from build123d import *


with BuildPart() as part:
    # Sketch5 → Revolve2 (revolve)
    with BuildSketch(Plane.XY):
        with BuildLine():
            ThreePointArc((6.647472776, -0.637932427), (6.425260177, 0.01668478), (6.35, 0.703880554))
            Line((6.35, 0.703880554), (6.35, 5.034871939))
            ThreePointArc((6.35, 5.034871939), (6.591682484, 6.249891837), (7.27993597, 7.27993597))
            Line((7.27993597, 7.27993597), (26.9875, 26.9875))
            Line((26.9875, 26.9875), (30.1625, 26.9875))
            Line((30.1625, 26.9875), (30.1625, -51.066071045))
            Line((30.1625, -51.066071045), (6.647472776, -0.637932427))
        make_face()
        with BuildLine():
            ThreePointArc((3.175, 5.034871939), (3.416682484, 6.249891837), (4.10493597, 7.27993597))
            Line((4.10493597, 7.27993597), (23.8125, 26.9875))
            Line((23.8125, 26.9875), (26.9875, 26.9875))
            Line((26.9875, 26.9875), (7.27993597, 7.27993597))
            ThreePointArc((7.27993597, 7.27993597), (6.591682484, 6.249891837), (6.35, 5.034871939))
            Line((6.35, 5.034871939), (6.35, 0.703880554))
            ThreePointArc((6.35, 0.703880554), (6.425260177, 0.01668478), (6.647472776, -0.637932427))
            Line((6.647472776, -0.637932427), (30.1625, -51.066071045))
            Line((30.1625, -51.066071045), (26.9875, -51.066071045))
            Line((26.9875, -51.066071045), (3.472472776, -0.637932427))
            ThreePointArc((3.472472776, -0.637932427), (3.250260177, 0.01668478), (3.175, 0.703880554))
            Line((3.175, 0.703880554), (3.175, 5.034871939))
        make_face()
    revolve(axis=Axis((0, 0, 0), (0, -1, 0)))


solid = part.part
Check sheet for the modelled part. Datum: model origin and axes. Units: mm. Give positions to 0.01 mm unless a question says otherwise; leave off trailing zeros. Write each loop counter-clockwise with the first axis right and the second up, starting at its lowest first coordinate (ties: lowest second). Pieces come first, ordered by that corner, then holes. Notation, with made-up numbers: (68.5, 35.25) -> (99.5, 35.25) arc R21 ccw to (99.5, 49.25) -> close; hole circle Ø4 at (52, -23). An arc over 180 degrees is marked (long way). One line per item, written item: value. Start each with the question number.
Item 1: Material ranges on probe 1 along Z at (x, y) = (0, 1) (1 decimal); probe 2 along Y at (x, z) = (-1, -13); probe 3 along Z at (x, y) = (-23, -20), recorded low to high. Write a range as from..to.
Item 2: Draft check along X on faces 1 (the cylindrical face through (-30.133, -12.586, 1.326)), 2 (the conical face through (-9.88, -19.9, -7.58)), 3 (the flat face through (22.2, 26.988, 9.1)). Enter one of: +X half, -X half, draft (parallel to the pull), parting line (faces both ways), or undercut.
Item 3: Section check C-C on y = -7. Record the cut outline in (x, z) (1 decimal).
Item 4: Gauge pin test, flat ends, axial feed: pin 1 (1 mm diameter, centred on y = -18.5, z = -14, fed in from -X); pin 2 (10 mm diameter, centred on x = 13, y = -32, fed in from -Z); pin 3 (12 mm diameter, centred on x = -11.5, z = 16.5, fed in from -Y). Record the tip position at first contact, or that the pin passes through.
Results list:
1. probe 1: -30.2..-3.2, 3.2..30.2
1. probe 2: -21.15..16.21
1. probe 3: -19.51..19.51
2. face 1: parting line
2. face 2: undercut
2. face 3: draft
3. outline: circle Ø60.3 at (0, 0); hole circle Ø12.9 at (0, 0)
4. pin 1: x = -26.97
4. pin 2: z = -29.08
4. pin 3: y = -49.19
